```python
from build123d import *

# Parameters (mm, degrees)
F0_R     = 6
F1_DEPTH = 10


with BuildPart() as f1:
    # F0 (on Front) → F1 (new body)
    with BuildSketch(Plane.XZ):
        with BuildLine():
            Line((35, 0), (29.859354, 52.901548))
            ThreePointArc((29.859354, 52.901548), (0, 80), (-29.859354, 52.901548))
            Line((-29.859354, 52.901548), (-35, 0))
            Line((-35, 0), (-60, 0))
            Line((-60, 0), (-60, -10))
            Line((-60, -10), (60, -10))
            Line((60, -10), (60, 0))
            Line((60, 0), (35, 0))
        make_face()
        with Locations((0, 50)):
            Circle(F0_R, mode=Mode.SUBTRACT)
    extrude(amount=F1_DEPTH)


solid = f1.part
```
Check sheet for the modelled part. Datum: model origin and axes. Units: mm. A direction names the side the tool comes from. Coordinates: 2 decimals unless noted, no trailing zeros. Order: outer loops, then holes, each group sorted by start corner. A loop starts at its lowest first (then second) coordinate and runs counter-clockwise, first axis right, second up. Notation, with made-up numbers: M 17,-32 L 51,-32 A12 ccw 51,-26 Z; hole C -29,20.5 d9. An arc over 180 degrees is marked long. Write each question's results on one line, items separated by ' | '. Start each with the question number.
1. Cross-section at C-C on z = 50. Record the cut outline in (x, y), and give its area (3 significant figures).
2. Cross-section at B-B on x = 0. Record the cut outline in (y, z), and give its area (3 significant figures).
3. Cross-section at D-D on x = -49.5. Record the cut outline in (y, z), and give its area (3 significant figures).
4. Go/stop test with flat-tipped pins: P1, Ø5, axis at x = -49, y = -3.5, coming from the +Z side; P2, Ø11, axis at x = 0, z = 50, coming from the -Y side; P3, Ø3, axis at y = -3.5, z = 69.5, coming from the +X side; P4, Ø6, axis at y = -5, z = 27, coming from the +X side. Record where each tip stops, or that it passes through.
5. Cross-section at A-A on y = -3. Record the cut outline in (x, z).
6. Mould release check, pull along X, two halves, no side actions. Record for faces 1 (the face through (-1.301, -4.93, 44.143)), 2 (the face through (-1, -10, 26)), 3 (the face through (0.619, -4.93, 79.994)): +X half, -X half, draft (parallel to the pull), parting line (faces both ways), or undercut.
7. Access from +Z, -Z, +X, -X, +Y, -Y to the whole of each face (thin tool, end or side, straight path). Record for faces 4 (the face through (48, -5, 0)), 5 (the face through (-60, -5, -5)), 6 (the face through (-47, -5, 0)).
8. Material ranges on probe 1 along Z at (x, y) = (0, -2); probe 2 along Z at (x, y) = (-5, -0.25); probe 3 along Z at (x, y) = (42, -8), recorded low to high.
Checks:
1) outline: M -30.14,-10 L -6,-10 L -6,0 L -30.14,0 Z; M 6,-10 L 30.14,-10 L 30.14,0 L 6,0 Z | area: 483 mm²
2) outline: M -10,-10 L 0,-10 L 0,44 L -10,44 Z; M -10,56 L 0,56 L 0,80 L -10,80 Z | area: 780 mm²
3) outline: M -10,-10 L 0,-10 L 0,0 L -10,0 Z | area: 100 mm²
4) P1: stops at z = 0 | P2: passes through | P3: stops at x = 24 | P4: stops at x = 32.67
5) outline: M -60,-10 L 60,-10 L 60,0 L 35,0 L 29.86,52.9 A30 ccw -29.86,52.9 L -35,0 L -60,0 Z; hole C 0,50 d12
6) face 1: undercut | face 2: draft | face 3: parting line
7) face 4: +Z, +X, +Y, -Y | face 5: +Z, -Z, -X, +Y, -Y | face 6: +Z, -X, +Y, -Y
8) probe 1: z = -10 to 44, 56 to 80 | probe 2: z = -10 to 46.68, 53.32 to 79.58 | probe 3: z = -10 to 0
